Build history of the part. All positions in model axes, mm. A direction names the side the tool comes from. Give positions to 0.01 mm unless a question says otherwise; leave off trailing zeros. Write each loop counter-clockwise with the first axis right and the second up, starting at its lowest first coordinate (ties: lowest second). Pieces come first, ordered by that corner, then holes.
from build123d import *

# Parameters (mm, degrees)
SKETCH_1_W          = 90
SKETCH_1_H          = 63
EXTRUDE_1_DEPTH     = 1
SKETCH_2_W          = 90
SKETCH_2_H          = 1
EXTRUDE_2_DEPTH     = 47
SKETCH_3_W          = 101.367565962
SKETCH_3_H          = 1
CUT_EXTRUDE_1_DEPTH = 31
SKETCH_4_W          = 31.251975893
SKETCH_4_H          = 48.889893619
SKETCH_4_W_2        = 31.654361849
CUT_EXTRUDE_2_DEPTH = 31
SKETCH_5_R          = 1.6
CUT_EXTRUDE_3_DEPTH = 31


with BuildPart() as part:
    # 草图1 → 凸台-拉伸1 (new body)
    with BuildSketch(Plane.XY):
        with Locations((45, 31.5)):
            Rectangle(SKETCH_1_W, SKETCH_1_H)
    extrude(amount=EXTRUDE_1_DEPTH)

    # 草图2 → 凸台-拉伸2 (add)
    with BuildSketch(Plane.XY.offset(1)):
        with Locations((45, 62.5)):
            Rectangle(SKETCH_2_W, SKETCH_2_H)
        with Locations((45, 0.5)):
            Rectangle(SKETCH_2_W, SKETCH_2_H)
    extrude(amount=EXTRUDE_2_DEPTH)

    # 草图3 → 切除-拉伸1 (cut)
    with BuildSketch(Plane.XY.offset(48)):
        with Locations((50.683782981, 0.5)):
            Rectangle(SKETCH_3_W, SKETCH_3_H)
    extrude(amount=-CUT_EXTRUDE_1_DEPTH, mode=Mode.SUBTRACT)

    # 草图4 → 切除-拉伸2 (cut)
    with BuildSketch(Plane.XY.offset(1)):
        with Locations((21.359825103, 30.997017556)):
            Rectangle(SKETCH_4_W, SKETCH_4_H)
        with Locations((64.951636971, 30.997017556)):
            Rectangle(SKETCH_4_W_2, SKETCH_4_H)
    extrude(amount=-CUT_EXTRUDE_2_DEPTH, mode=Mode.SUBTRACT)

    # 草图5 → 切除-拉伸3 (cut)
    with BuildSketch(Plane.XZ.offset(-62)):
        with Locations(Location((8.358150818, 38, 0), (0, 0, 270))):
            Circle(SKETCH_5_R)
        with Locations(Location((82.205212472, 38, 0), (0, 0, 270))):
            Circle(SKETCH_5_R)
    extrude(amount=-CUT_EXTRUDE_3_DEPTH, mode=Mode.SUBTRACT)


solid = part.part
(1) Mould opens along Y. For faces 1 (the face through (44, 1, 9)), 2 (the face through (44, 32, 0)), 3 (the face through (44, 32, 1)), 4 (the face through (44, 0, 8)) say: +Y half, -Y half, draft (parallel to the pull), parting line (faces both ways), or undercut.
(2) Drop flat-ended pins along their axis: pin 1 (0.8 mm diameter, centred on x = 44.5, y = 0.5, fed in from +Z); pin 2 (3 mm diameter, centred on x = 82.21, z = 38, fed in from -Y); pin 3 (8 mm diameter, centred on x = 39.5, y = 13.5, fed in from +Z). Give the stop position or say it passes through.
(3) Saw through at C-C, the plane y = 31. List the corners of the cut face in (x, z).
(4) Saw through at A-A, the plane x = 78. List the corners of the cut face in (y, z).
(5) Saw through at D-D, the plane x = 39.5. List the corners of the cut face in (y, z), plus the area to 3 significant figures.
(6) Probe line 1 (Y direction, x = 40.5, z = 2); line 2 (Y direction, x = 62, z = 33); line 3 (Z direction, x = 11, y = 55.5). List the from-to ranges inside material, lowest first.
(7) Saw through at B-B, the plane z = 38. List the corners of the cut face in (x, y).
(8) 3-axis set-ups, long thin cutter, end or side, ignore diameter. For faces 5 (the face through (44, 62, 24)), 6 (the face through (9.44, 62.49, 39.18)): which of +Z, -Z, +X, -X, +Y, -Y reach the whole face in a straight line?
Computed values:
1. face 1: undercut
1. face 2: draft
1. face 3: undercut
1. face 4: -Y half
2. pin 1: stops at z = 17
2. pin 2: passes through
2. pin 3: stops at z = 1
3. outline: (0, 0) - (5.73, 0) - (5.73, 1) - (0, 1) - close; (36.99, 0) - (49.12, 0) - (49.12, 1) - (36.99, 1) - close; (80.78, 0) - (90, 0) - (90, 1) - (80.78, 1) - close
4. outline: (0, 0) - (6.55, 0) - (6.55, 1) - (1, 1) - (1, 17) - (0, 17) - close; (55.44, 0) - (63, 0) - (63, 48) - (62, 48) - (62, 1) - (55.44, 1) - close
5. outline: (0, 0) - (63, 0) - (63, 48) - (62, 48) - (62, 1) - (1, 1) - (1, 17) - (0, 17) - close
5. area: 126 mm2
6. line 1: y = 0 to 1, 62 to 63
6. line 2: y = 62 to 63
6. line 3: z = 0 to 1
7. outline: (0, 62) - (6.76, 62) - (6.76, 63) - (0, 63) - close; (9.96, 62) - (80.61, 62) - (80.61, 63) - (9.96, 63) - close; (83.81, 62) - (90, 62) - (90, 63) - (83.81, 63) - close
8. face 5: +Z, +X, -X
8. face 6: +Y, -Y
